Job drawing, mm, ordinate dimensions from the low corner. One solid piece. A direction names the side the tool comes from. Give positions to 0.01 mm unless a question says otherwise; leave off trailing zeros. Write each loop counter-clockwise with the first axis right and the second up, starting at its lowest first coordinate (ties: lowest second). Pieces come first, ordered by that corner, then holes. Notation, with made-up numbers: M -14,14 L -5,14 A20 ccw -5,26 Z; hole C 29.25,33.25 d8. An arc over 180 degrees is marked long. Answer as CSV lines item,"result". Start each with the question number.
1) Slice it at B-B, the plane y = 1.75. Give the cut face in (x, z), plus the area to 3 significant figures.
2) Slice it at A-A, the plane z = 5.25. Give the cut face in (x, y), plus the area to 3 significant figures.
3) Pin check, flat tips, straight feed: pin 1 Ø3 at (x, z) = (1, 4) entering from -Y; pin 2 Ø1 at (x, z) = (4, 4) entering from -Y; pin 3 Ø1 at (x, y) = (4, 3) entering from +Z. Stop position of each tip, or through.
4) Tool access for the marked faces 4 and 5: list every direction of +Z, -Z, +X, -X, +Y, -Y with a clear straight run to the whole face (end or side of a thin tool).
5) Mould opens along X. For the marked faces 1, 2 and 3 say: pulls with the +X half, pulls with the -X half, needs draft (parallel to the pull), parting line crosses it, or undercut.
6) Wall check: line 1 along X through (y, z) = (2.75, 5.15); line 2 along Y through (x, z) = (2, 4.8); line 3 along Z through (x, y) = (4.75, 0.5). Give the ranges that are in metal, low to high. Write a range as from..to.
7) Slice it at C-C, the plane x = 4.75. Give the cut face in (y, z).
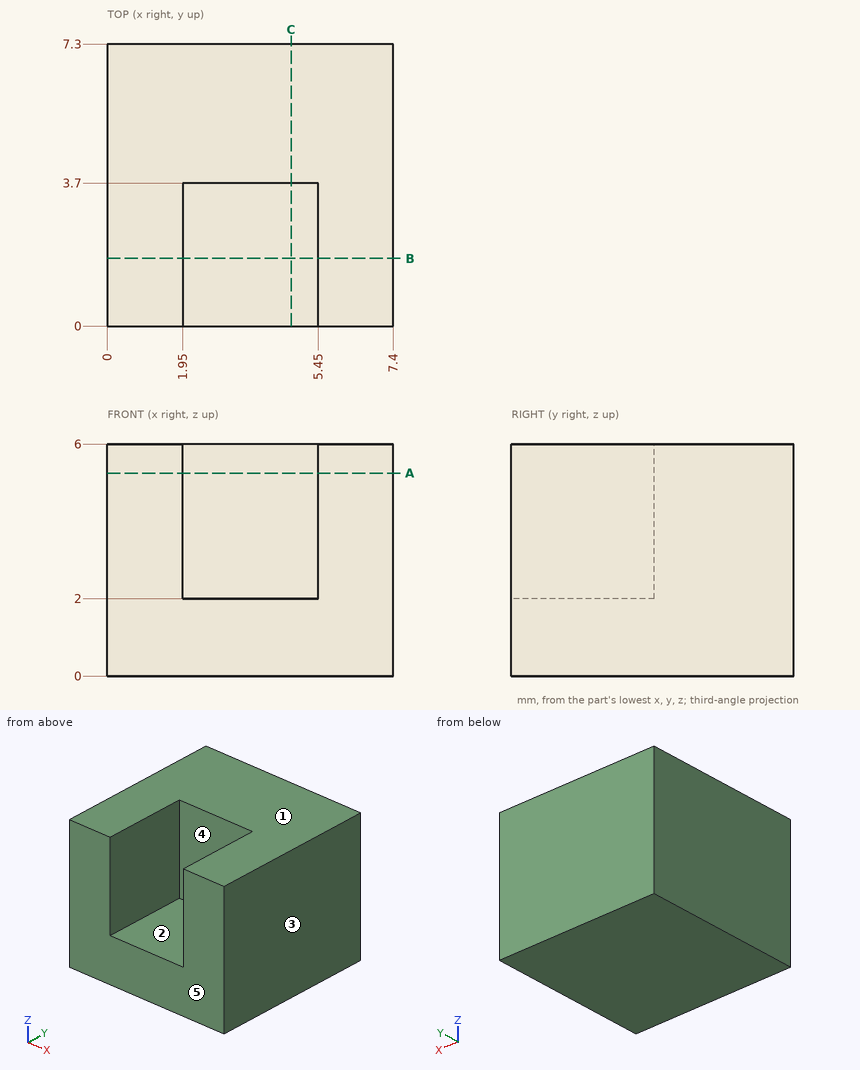
Found:
1,outline,"M 0,0 L 7.4,0 L 7.4,6 L 5.45,6 L 5.45,2 L 1.95,2 L 1.95,6 L 0,6 Z"
1,area,"30.4 mm²"
2,outline,"M 0,0 L 1.95,0 L 1.95,3.7 L 5.45,3.7 L 5.45,0 L 7.4,0 L 7.4,7.3 L 0,7.3 Z"
2,area,"41.1 mm²"
3,pin 1,"y = 0"
3,pin 2,"y = 3.7"
3,pin 3,"z = 2"
4,face 4,"+Z, -Y"
4,face 5,"+Z, -Z, +X, -X, -Y"
5,face 1,"needs draft"
5,face 2,"undercut"
5,face 3,"pulls with the +X half"
6,line 1,"0..1.95, 5.45..7.4"
6,line 2,"3.7..7.3"
6,line 3,"0..2"
7,outline,"M 0,0 L 7.3,0 L 7.3,6 L 3.7,6 L 3.7,2 L 0,2 Z"
